The model under review builds one solid part; all positions refer to its coordinate system, in mm. Round coordinates to 2 decimals unless told otherwise and drop trailing zeros. Write each loop counter-clockwise with the first axis right and the second up, starting at its lowest first coordinate (ties: lowest second). Pieces come first, ordered by that corner, then holes. Notation, with made-up numbers: (50, -10) - (79, -10) arc R27 ccw to (79, 16) - close; hole circle Ø11 at (83.5, 73.25). An arc over 180 degrees is marked (long way). Use one line per item in the form item = value.
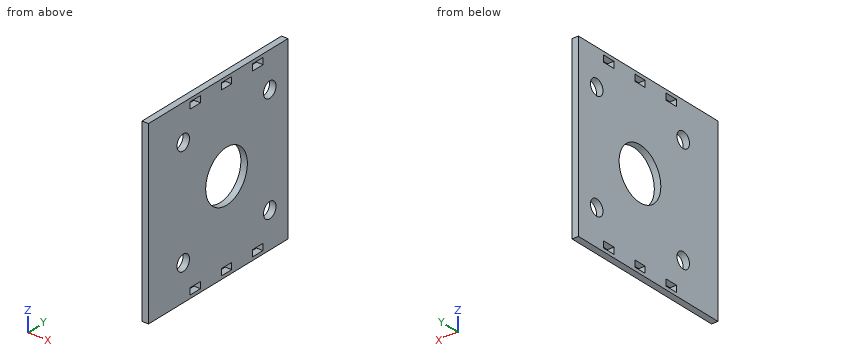
from build123d import *

# Parameters (mm, degrees)
SKETCH4_R           = 6
SKETCH4_R_2         = 20
SKETCH4_W           = 5
SKETCH4_H           = 9.999474932
BOSS_EXTRUDE2_DEPTH = 5


with BuildPart() as part:
    # Sketch4 → Boss-Extrude2 (new body)
    with BuildSketch(Plane(origin=(0, 0, 0), x_dir=(0, 0, -1), z_dir=(1, 0, 0))):
        Polygon((-59, 59), (59, 59), (69, 59), (69, -59), (69, -74.875), (-69, -74.875), (-69, -59), (-69, 59), align=None)
        with Locations((41.5, 41.5)):
            Circle(SKETCH4_R, mode=Mode.SUBTRACT)
        with Locations((41.5, -41.5)):
            Circle(SKETCH4_R, mode=Mode.SUBTRACT)
        with Locations((-41.5, 41.5)):
            Circle(SKETCH4_R, mode=Mode.SUBTRACT)
        with Locations((-41.5, -41.5)):
            Circle(SKETCH4_R, mode=Mode.SUBTRACT)
        Circle(SKETCH4_R_2, mode=Mode.SUBTRACT)
        with Locations((-64, 0)):
            Rectangle(SKETCH4_W, SKETCH4_H, mode=Mode.SUBTRACT)
        with Locations((-64, 30)):
            Rectangle(SKETCH4_W, SKETCH4_H, mode=Mode.SUBTRACT)
        with Locations((-64, -30)):
            Rectangle(SKETCH4_W, SKETCH4_H, mode=Mode.SUBTRACT)
        with Locations((64, 30)):
            Rectangle(SKETCH4_W, SKETCH4_H, mode=Mode.SUBTRACT)
        with Locations((64, 0)):
            Rectangle(SKETCH4_W, SKETCH4_H, mode=Mode.SUBTRACT)
        with Locations((64, -30)):
            Rectangle(SKETCH4_W, SKETCH4_H, mode=Mode.SUBTRACT)
    extrude(amount=BOSS_EXTRUDE2_DEPTH)


solid = part.part
(1) Add section C-C on z = 0. Write out the cut boundary in (x, y) (3 decimals).
Geometry results:
outline = (0, -74.875) - (5, -74.875) - (5, -20) - (0, -20) - close; (0, 20) - (5, 20) - (5, 59) - (0, 59) - close
(2) Insertion check: P1, Ø11, axis at y = -41.5, z = -41.5, coming from the +X side. The pin has a flat end and moves straight along its axis. Give the tip position at first contact, or say it passes through.
Geometry results:
P1 = through
(3) Add section D-D on x = 1.85. Count the separate pieces of the cut face and the enclosed holes in it, then the cut area to 3 significant figures.
Geometry results:
separate_pieces = 1
enclosed_holes = 11
area = 16,500 mm2
(4) Add section A-A on z = -41.5. Write out the cut boundary in (x, y) (3 decimals).
Geometry results:
outline = (0, -74.875) - (5, -74.875) - (5, -47.5) - (0, -47.5) - close; (0, -35.5) - (5, -35.5) - (5, 35.5) - (0, 35.5) - close; (0, 47.5) - (5, 47.5) - (5, 59) - (0, 59) - close
(5) To check wall thickness, follow L1, parallel to Y at x = 1.65, z = -41.5 (3 decimals); L2, parallel to Z at x = 0.7, y = -3; L3, parallel to Y at x = 3.5, z = 36.5 (3 decimals). State the ranges of each line that lie inside material, in increasing order.
Geometry results:
L1 = -74.875 to -47.5, -35.5 to 35.5, 47.5 to 59
L2 = -69 to -66.5, -61.5 to -19.77, 19.77 to 61.5, 66.5 to 69
L3 = -74.875 to -44.817, -38.183 to 38.183, 44.817 to 59
(6) Add section B-B on y = 41.5. Write out the cut boundary in (x, z), then the cut area to 3 significant figures.
Geometry results:
outline = (0, -69) - (5, -69) - (5, -47.5) - (0, -47.5) - close; (0, -35.5) - (5, -35.5) - (5, 35.5) - (0, 35.5) - close; (0, 47.5) - (5, 47.5) - (5, 69) - (0, 69) - close
area = 570 mm2
